Autodesk Inventor part; units mm, degrees
ref_plane "YZ Plane" through (0, 0, 0) normal (1, 0, 0) x (0, 1, 0)
ref_plane "XZ Plane" through (0, 0, 0) normal (0, 1, 0) x (-1, 0, 0)
ref_plane "XY Plane" through (0, 0, 0) normal (0, 0, 1) x (1, 0, 0)
sketch "Sketch1" plane through (0, 0, 0) normal (0, 1, 0) x (-1, 0, 0)
  line L0 (3.175, 0) -> (17.653, 0)
  line L1 (20.828, -3.175) -> (20.828, -17.145)
  line L2 (17.653, -20.32) -> (3.175, -20.32)
  line L3 (0, -17.145) -> (0, -3.175)
  circle A0 centre (2.6416, -2.5146) radius 1.2446
  circle A1 centre (2.6416, -17.8054) radius 1.2446
  line L4 (1.397, -2.5146) -> (0, -2.5146) construction
  line L5 (2.6416, -1.27) -> (2.6416, 0) construction
  line L6 (1.397, -17.8054) -> (0, -17.8054) construction
  line L7 (2.6416, -19.05) -> (2.6416, -20.32) construction
  arc A2 (0, -17.145) -> (3.175, -20.32) centre (3.175, -17.145) ccw
  arc A3 (3.175, 0) -> (0, -3.175) centre (3.175, -3.175) ccw
  arc A4 (20.828, -3.175) -> (17.653, 0) centre (17.653, -3.175) ccw
  arc A5 (17.653, -20.32) -> (20.828, -17.145) centre (17.653, -17.145) ccw
  point P0 (0, 0)
  point P1 (20.828, -20.32)
  point P2 (20.828, 0)
  point P3 (0, -20.32)
  dimension "d0" = 20.32
  dimension "d1" = 20.828
  dimension "d2" = 2.4892
  dimension "d3" = 2.4892
  dimension "d4" = 1.397
  dimension "d5" = 1.27
  dimension "d6" = 1.27
  dimension "d7" = 1.397
  dimension "d8" = 3.175
extrude "Extrusion1" add sketch "Sketch1" along normal blind 1.651
sketch "Sketch2" plane through (0, 1.651, 0) normal (0, 1, 0) x (1, 0, 0)
  line L0 (-11.557, 9.017) -> (-9.271, 9.017)
  line L1 (-9.271, 9.017) -> (-9.271, 11.303)
  line L2 (-9.271, 11.303) -> (-11.557, 11.303)
  line L3 (-11.557, 11.303) -> (-11.557, 9.017)
  line L4 (-11.557, 10.16) -> (-9.271, 10.16) construction
  line L5 (-10.414, 9.017) -> (-10.414, 11.303) construction
  line L6 (-3.175, 20.32) -> (-17.653, 20.32)
  line L7 (-20.828, 17.145) -> (-20.828, 3.175)
  point P0 (0, 0)
  point P1 (-10.414, 20.32)
  point P2 (-20.828, 10.16)
  dimension "d11" = 2.286
  dimension "d12" = 2.286
extrude "Extrusion2" add sketch "Sketch2" along normal blind 0.5842
sketch "Sketch3" plane through (0, 0, 0) normal (0, -1, 0) x (1, 0, 0)
  line L0 (-18.3896, -19.431) -> (-17.6022, -19.431)
  line L1 (-16.8402, -18.669) -> (-16.8402, -1.651)
  line L2 (-17.6022, -0.889) -> (-18.3896, -0.889)
  line L3 (-19.1516, -1.651) -> (-19.1516, -18.669)
  line L4 (-17.653, -20.32) -> (-3.175, -20.32)
  line L5 (-3.175, 0) -> (-17.653, 0)
  line L6 (-20.828, -3.175) -> (-20.828, -17.145)
  arc A0 (-19.1516, -18.669) -> (-18.3896, -19.431) centre (-18.3896, -18.669) ccw
  arc A1 (-18.3896, -0.889) -> (-19.1516, -1.651) centre (-18.3896, -1.651) ccw
  arc A2 (-16.8402, -1.651) -> (-17.6022, -0.889) centre (-17.6022, -1.651) ccw
  arc A3 (-17.6022, -19.431) -> (-16.8402, -18.669) centre (-17.6022, -18.669) ccw
  point P0 (0, 0)
  dimension "d15" = 0.889
  dimension "d16" = 0.889
  dimension "d17" = 3.9878
  dimension "d18" = 1.6764
  dimension "d19" = 0.762
extrude "Extrusion3" add sketch "Sketch3" along normal blind 2.54
sketch "Sketch4" plane through (0, -2.54, 0) normal (0, -1, 0) x (1, 0, 0)
  line L0 (-18.415, -17.6657) -> (-17.5768, -17.6657)
  line L1 (-17.5768, -17.6657) -> (-17.5768, -16.8275)
  line L2 (-17.5768, -16.8275) -> (-18.415, -16.8275)
  line L3 (-18.415, -16.8275) -> (-18.415, -17.6657)
  line L4 (-17.9959, -17.6657) -> (-17.9959, -16.8275) construction
  line L5 (-18.3896, -19.431) -> (-17.6022, -19.431)
  line L6 (-18.415, -15.3035) -> (-17.5768, -15.3035)
  line L7 (-17.5768, -15.3035) -> (-17.5768, -14.4653)
  line L8 (-17.5768, -14.4653) -> (-18.415, -14.4653)
  line L9 (-18.415, -14.4653) -> (-18.415, -15.3035)
  line L10 (-17.9959, -15.3035) -> (-17.9959, -14.4653) construction
  line L11 (-18.415, -12.9413) -> (-17.5768, -12.9413)
  line L12 (-17.5768, -12.9413) -> (-17.5768, -12.1031)
  line L13 (-17.5768, -12.1031) -> (-18.415, -12.1031)
  line L14 (-18.415, -12.1031) -> (-18.415, -12.9413)
  line L15 (-17.9959, -12.9413) -> (-17.9959, -12.1031) construction
  line L16 (-18.415, -10.5791) -> (-17.5768, -10.5791)
  line L17 (-17.5768, -10.5791) -> (-17.5768, -9.7409)
  line L18 (-17.5768, -9.7409) -> (-18.415, -9.7409)
  line L19 (-18.415, -9.7409) -> (-18.415, -10.5791)
  line L20 (-17.9959, -10.5791) -> (-17.9959, -9.7409) construction
  line L21 (-18.415, -8.2169) -> (-17.5768, -8.2169)
  line L22 (-17.5768, -8.2169) -> (-17.5768, -7.3787)
  line L23 (-17.5768, -7.3787) -> (-18.415, -7.3787)
  line L24 (-18.415, -7.3787) -> (-18.415, -8.2169)
  line L25 (-17.9959, -8.2169) -> (-17.9959, -7.3787) construction
  line L26 (-18.415, -5.8547) -> (-17.5768, -5.8547)
  line L27 (-17.5768, -5.8547) -> (-17.5768, -5.0165)
  line L28 (-17.5768, -5.0165) -> (-18.415, -5.0165)
  line L29 (-18.415, -5.0165) -> (-18.415, -5.8547)
  line L30 (-17.9959, -5.8547) -> (-17.9959, -5.0165) construction
  line L31 (-18.415, -3.4925) -> (-17.5768, -3.4925)
  line L32 (-17.5768, -3.4925) -> (-17.5768, -2.6543)
  line L33 (-17.5768, -2.6543) -> (-18.415, -2.6543)
  line L34 (-18.415, -2.6543) -> (-18.415, -3.4925)
  line L35 (-17.9959, -3.4925) -> (-17.9959, -2.6543) construction
  line L36 (-18.415, -10.16) -> (-17.5768, -10.16) construction
  line L37 (-19.1516, -1.651) -> (-19.1516, -18.669)
  point P0 (0, 0)
  point P1 (-17.9959, -19.431)
  point P2 (-17.9959, -17.0688)
  point P3 (-17.9959, -14.7066)
  point P4 (-17.9959, -12.3444)
  point P5 (-17.9959, -9.9822)
  point P6 (-17.9959, -7.62)
  point P7 (-17.9959, -5.2578)
  point P8 (-19.1516, -10.16)
  dimension "d22" = 0.8382
  dimension "d23" = 0.8382
  dimension "d26" = 2.3622
extrude "Extrusion4" add sketch "Sketch4" along normal blind 5.842
chamfer "Chamfer1" distance 0.254 angle 45 28 edges at (-18.415, -8.382, -17.2466) (-17.9959, -8.382, -17.6657) (-17.5768, -8.382, -17.2466) (-17.9959, -8.382, -16.8275) (-18.415, -8.382, -14.8844) (-17.9959, -8.382, -15.3035) (-17.5768, -8.382, -14.8844) (-17.9959, -8.382, -14.4653) (-17.9959, -8.382, -12.9413) (-18.415, -8.382, -12.5222) (-17.9959, -8.382, -12.1031) (-17.5768, -8.382, -12.5222) (-17.5768, -8.382, -10.16) (-17.9959, -8.382, -9.7409) (-18.415, -8.382, -10.16) (-17.9959, -8.382, -10.5791) (-17.9959, -8.382, -8.2169) (-18.415, -8.382, -7.7978) (-17.9959, -8.382, -7.3787) (-17.5768, -8.382, -7.7978) (-18.415, -8.382, -5.4356) (-17.9959, -8.382, -5.0165) (-17.5768, -8.382, -5.4356) (-17.9959, -8.382, -5.8547) (-17.9959, -8.382, -3.4925) (-18.415, -8.382, -3.0734) (-17.9959, -8.382, -2.6543) (-17.5768, -8.382, -3.0734)
equation "\"d3\" = d2"
equation "\"d6\" = d5"
equation "\"d7\" = d4"
properties part number "Adafruit TMP007 IR Sensor"
Source: CAD feature listing. Evaluate the final solid. Frame: model axes, mm. A direction names the side the tool comes from. Give positions to 0.01 mm unless a question says otherwise; leave off trailing zeros. Write each loop counter-clockwise with the first axis right and the second up, starting at its lowest first coordinate (ties: lowest second). Pieces come first, ordered by that corner, then holes.
1. Section query B-B (y = 1). Return the cut outline in (x, z) (3 decimals).
2. Section query C-C (z = -2). Return the cut outline in (x, y).
3. Material intervals for line 1 along X through (y, z) = (-0.5, -13); line 2 along Y through (x, z) = (-1.25, -3.75); line 3 along X through (y, z) = (-4.75, -7.75) (3 decimals), sorted ascending.
4. Access query for faces 5 (the face through (-17.577, -5, -17)), 6 (the face through (-18, -5, -10.579)), 7 (the face through (-19.152, -1, -10)). Directions: +Z, -Z, +X, -X, +Y, -Y. A direction counts if a zero-diameter tool reaches every point of the face in a straight line with its end or side. Return the directions, or none.
5. First-contact query: pin 1 (0.9 mm diameter, centred on y = -6.5, z = -10, fed in from -X) (3 decimals); pin 2 (0.7 mm diameter, centred on x = -18, y = -4, fed in from -Z); pin 3 (3 mm diameter, centred on x = -11.5, z = -15, fed in from +Y); pin 4 (5 mm diameter, centred on x = -16.5, y = -2, fed in from +Z). Flat tips, straight axial feed; report the tip coordinate or a pass-through.
6. Section query D-D (x = -1.75). Return the cut outline in (y, z).
7. Section query A-A (y = -4.75). Return the cut outline in (x, z) (1 decimal).
8. Pull-direction query (X, two-part tool) for faces 1 (the face through (-17.577, -5, -3)), 2 (the face through (-2.37, 0.81, -16.59)), 3 (the face through (-19, -2.54, -10)), 4 (the face through (-20.828, 1, -10)); classes: +X half, -X half, draft (parallel to the pull), parting line (faces both ways), or undercut.
Output values:
1. outline: (-20.828, -17.145) arc R3.175 ccw to (-17.653, -20.32) - (-3.175, -20.32) arc R3.175 ccw to (0, -17.145) - (0, -3.175) arc R3.175 ccw to (-3.175, 0) - (-17.653, 0) arc R3.175 ccw to (-20.828, -3.175) - close; hole circle Ø2.489 at (-2.642, -17.805); hole circle Ø2.489 at (-2.642, -2.515)
2. outline: (-20.6, 0) - (-19.15, 0) - (-19.15, -2.54) - (-16.84, -2.54) - (-16.84, 0) - (-3.77, 0) - (-3.77, 1.65) - (-20.6, 1.65) - close; (-1.51, 0) - (-0.23, 0) - (-0.23, 1.65) - (-1.51, 1.65) - close
3. line 1: x = -19.15 to -16.84
3. line 2: y = 0 to 1.65
3. line 3: x = -18.415 to -17.577
4. face 5: +Z, -Z, +X, -Y
4. face 6: +X, -X, -Y
4. face 7: +Z, -Z, -X, -Y
5. pin 1: stops at x = -18.415
5. pin 2: stops at z = -17.67
5. pin 3: stops at y = 1.65
5. pin 4: stops at z = 0
6. outline: (0, -19.98) - (1.65, -19.98) - (1.65, -18.67) - (0, -18.67) - close; (0, -16.94) - (1.65, -16.94) - (1.65, -3.38) - (0, -3.38) - close; (0, -1.65) - (1.65, -1.65) - (1.65, -0.34) - (0, -0.34) - close
7. outline: (-18.4, -17.7) - (-17.6, -17.7) - (-17.6, -16.8) - (-18.4, -16.8) - close; (-18.4, -15.3) - (-17.6, -15.3) - (-17.6, -14.5) - (-18.4, -14.5) - close; (-18.4, -12.9) - (-17.6, -12.9) - (-17.6, -12.1) - (-18.4, -12.1) - close; (-18.4, -10.6) - (-17.6, -10.6) - (-17.6, -9.7) - (-18.4, -9.7) - close; (-18.4, -8.2) - (-17.6, -8.2) - (-17.6, -7.4) - (-18.4, -7.4) - close; (-18.4, -5.9) - (-17.6, -5.9) - (-17.6, -5) - (-18.4, -5) - close; (-18.4, -3.5) - (-17.6, -3.5) - (-17.6, -2.7) - (-18.4, -2.7) - close
8. face 1: +X half
8. face 2: undercut
8. face 3: draft
8. face 4: -X half
